Source: CAD feature listing. Evaluate the final solid. Frame: model axes, mm. Face numbers are marked on the shaded views. A direction names the side the tool comes from. Round coordinates to 2 decimals unless told otherwise and drop trailing zeros. Order: outer loops, then holes, each group sorted by start corner. A loop starts at its lowest first (then second) coordinate and runs counter-clockwise, first axis right, second up. Notation, with made-up numbers: (43, 15.25) - (57, 15.25) arc R11 ccw to (57, 23.25) - close; hole circle Ø8 at (3, 75.5). An arc over 180 degrees is marked (long way). Put each result on its own line as item: value. Start each with the question number.
1) Contact query for flat-ended pins moving along their axis: P1, Ø6, axis at x = 68, z = -49.5, coming from the +Y side; P2, Ø4.5, axis at y = -44.5, z = 65, coming from the +X side; P3, Ø5, axis at y = 34, z = 47.5, coming from the -X side; P4, Ø5, axis at x = 10, y = -28, coming from the +Z side. Output: stop coordinate, or through.
2) Line query: probe 1 along Y at (x, z) = (1.5, -30); probe 2 along Y at (x, z) = (90.5, -23.5); probe 3 along Z at (x, y) = (1, -51). Output: solid intervals per line, ascending. Write a range as [from, to].
3) Section A-A on x = -7. Output: boundary loops of the cut face in (y, z).
4) Section B-B on z = 0. Output: boundary loops of the cut face in (x, y).
5) Section D-D on x = 38.5. Output: boundary loops of the cut face in (y, z), then the cut area to 3 significant figures.
6) Access query for the marked faces 4, 5 and 6. Directions: +Z, -Z, +X, -X, +Y, -Y. A direction counts if a zero-diameter tool reaches every point of the face in a straight line with its end or side. Return the directions, or none.
7) Section C-C on z = -21. Output: boundary loops of the cut face in (x, y), then the cut area to 3 significant figures.
8) Mould query, pull axis Z, two halves, no side actions, for the marked faces 1, 2 and 3. Classes: +Z half, -Z half, draft (parallel to the pull), parting line (faces both ways), or undercut.
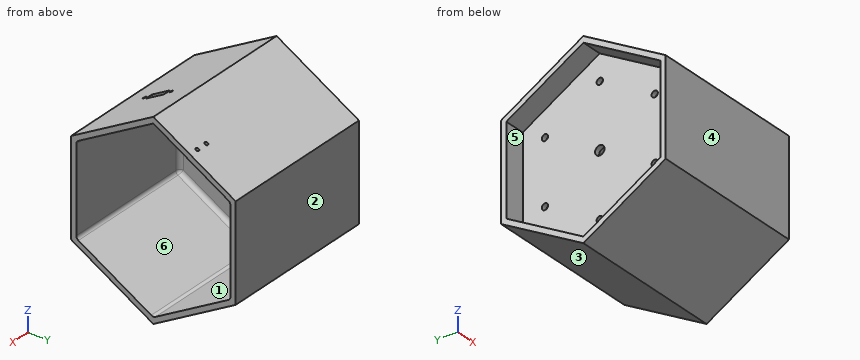
```python
from build123d import *

# Parameters (mm, degrees)
BOSS_EXTRUDE1_DEPTH = 200
CUT_EXTRUDE1_DEPTH  = 195
SKETCH5_R           = 1.65
SKETCH5_W           = 7.65
SKETCH5_H           = 20.2
CUT_EXTRUDE4_DEPTH  = 70
SKETCH7_R           = 4.5
SKETCH7_R_2         = 3
CUT_EXTRUDE6_DEPTH  = 70
FILLET1_R           = 4
CUT_EXTRUDE7_DEPTH  = 70
SKETCH10_R          = 1.6
CUT_EXTRUDE8_DEPTH  = 6
BOSS_EXTRUDE2_DEPTH = 20


with BuildPart() as part:
    # Sketch1 → Boss-Extrude1 (new body)
    with BuildSketch(Plane(origin=(0, 0, 0), x_dir=(0, 0, -1), z_dir=(1, 0, 0))):
        Polygon((90, 0), (45, 77.942286341), (-45, 77.942286341), (-90, 0), (-45, -77.942286341), (45, -77.942286341), align=None)
    extrude(amount=BOSS_EXTRUDE1_DEPTH)

    # Sketch2 → Cut-Extrude1 (cut)
    with BuildSketch(Plane(origin=(200, 0, 0), x_dir=(0, 0, -1), z_dir=(1, 0, 0))):
        Polygon((84.226497308, 0), (42.113248654, 72.942286341), (-42.113248654, 72.942286341), (-84.226497308, 0), (-42.113248654, -72.942286341), (42.113248654, -72.942286341), align=None)
    extrude(amount=-CUT_EXTRUDE1_DEPTH, mode=Mode.SUBTRACT)

    # Sketch5 → Cut-Extrude4 (cut)
    with BuildSketch(Plane(origin=(0, -38.97114317, 67.5), x_dir=(1, 0, 0), z_dir=(0, -0.500000000000007, 0.8660254037844347))):
        with Locations(Location((68.825, 9.75, 0), (0, 0, 270))):
            Circle(SKETCH5_R)
        with Locations(Location((68.825, -19.75, 0), (0, 0, 270))):
            Circle(SKETCH5_R)
        with Locations((68.825, -5)):
            Rectangle(SKETCH5_W, SKETCH5_H)
    extrude(amount=-CUT_EXTRUDE4_DEPTH, mode=Mode.SUBTRACT)

    # Sketch7 → Cut-Extrude6 (cut)
    with BuildSketch(Plane(origin=(5, 0, 0), x_dir=(0, 0, -1), z_dir=(1, 0, 0))):
        Circle(SKETCH7_R)
        with Locations((60, 0)):
            Circle(SKETCH7_R_2)
        with Locations((30, 51.961524227)):
            Circle(SKETCH7_R_2)
        with Locations((-30, 51.961524227)):
            Circle(SKETCH7_R_2)
        with Locations((-60, 0)):
            Circle(SKETCH7_R_2)
        with Locations((-30, -51.961524227)):
            Circle(SKETCH7_R_2)
        with Locations((30, -51.961524227)):
            Circle(SKETCH7_R_2)
    extrude(amount=-CUT_EXTRUDE6_DEPTH, mode=Mode.SUBTRACT)

    # Fillet1
    fillet1_edges = [part.edges().sort_by_distance(p)[0] for p in [
        (5, -36.47114317, -63.169872981),
        (102.5, 0, -84.226497308),
        (5, -72.942286341, 0),
        (102.5, -72.942286341, -42.113248654),
        (5, -36.47114317, 63.169872981),
        (102.5, -72.942286341, 42.113248654),
        (5, 36.47114317, 63.169872981),
        (5, 72.942286341, 0),
        (102.5, 72.942286341, 42.113248654),
        (5, 36.47114317, -63.169872981),
        (102.5, 72.942286341, -42.113248654),
    ]]
    fillet(fillet1_edges, radius=FILLET1_R)

    # Sketch9 → Cut-Extrude7 (cut)
    with BuildSketch(Plane(origin=(200, 0, 0), x_dir=(0, 0, -1), z_dir=(1, 0, 0))):
        Polygon((45, 77.942286341), (90, 0), (45, -77.942286341), (-45, -77.942286341), (-90, 0), (-45, 77.942286341), align=None)
    extrude(amount=-CUT_EXTRUDE7_DEPTH, mode=Mode.SUBTRACT)

    # Sketch10 → Cut-Extrude8 (cut)
    with BuildSketch(Plane(origin=(0, 38.97114317, 67.5), x_dir=(1, 0, 0), z_dir=(0, 0.49999999999999495, 0.8660254037844417))):
        with Locations(Location((110, -5, 0), (0, 0, 270))):
            Circle(SKETCH10_R)
        with Locations(Location((121, -5, 0), (0, 0, 270))):
            Circle(SKETCH10_R)
    extrude(amount=-CUT_EXTRUDE8_DEPTH, mode=Mode.SUBTRACT)

    # Sketch11 → Boss-Extrude2 (add)
    with BuildSketch(Plane.ZY):
        Polygon((90, 0), (45, 77.942286341), (-45, 77.942286341), (-90, 0), (-45, -77.942286341), (45, -77.942286341), align=None)
        Polygon((84.226497308, 0), (42.113248654, 72.942286341), (-42.113248654, 72.942286341), (-84.226497308, 0), (-42.113248654, -72.942286341), (42.113248654, -72.942286341), align=None, mode=Mode.SUBTRACT)
    extrude(amount=BOSS_EXTRUDE2_DEPTH)


solid = part.part
```
Answer sheet:
1. P1: y = 75.34
1. P2: x = 130
1. P3: x = 0
1. P4: z = 75.28
2. probe 1: [-77.94, -54.96], [-48.96, 48.96], [54.96, 77.94]
2. probe 2: [-77.94, -72.94], [72.94, 77.94]
2. probe 3: [-60.56, -32.84], [-27.16, 27.16], [32.84, 60.56]
3. outline: (-77.94, -45) - (0, -90) - (77.94, -45) - (77.94, 45) - (0, 90) - (-77.94, 45) - close; hole (-72.94, -42.11) - (0, -84.23) - (72.94, -42.11) - (72.94, 42.11) - (0, 84.23) - (-72.94, 42.11) - close
4. outline: (-20, -77.94) - (130, -77.94) - (130, -72.94) - (9, -72.94) arc R4 cw to (5, -68.94) - (5, -4.5) - (0, -4.5) - (0, -72.94) - (-20, -72.94) - close; (-20, 72.94) - (0, 72.94) - (0, 4.5) - (5, 4.5) - (5, 68.94) arc R4 cw to (9, 72.94) - (130, 72.94) - (130, 77.94) - (-20, 77.94) - close
5. outline: (-77.94, -45) - (0, -90) - (77.94, -45) - (77.94, 45) - (0, 90) - (-77.94, 45) - close; hole (-72.94, -39.8) arc R4 ccw to (-70.94, -43.27) - (-2, -83.07) arc R4 ccw to (2, -83.07) - (70.94, -43.27) arc R4 ccw to (72.94, -39.8) - (72.94, 39.8) arc R4 ccw to (70.94, 43.27) - (0, 84.23) - (-70.94, 43.27) arc R4 ccw to (-72.94, 39.8) - close
5. area: 2,620 mm^2
6. face 4: +Z, -Z, +X, -X, -Y
6. face 5: -X
6. face 6: +X
7. outline: (-20, -77.94) - (130, -77.94) - (130, -72.94) - (9, -72.94) arc R4 cw to (5, -68.94) - (5, 68.94) arc R4 cw to (9, 72.94) - (130, 72.94) - (130, 77.94) - (-20, 77.94) - (-20, 72.94) - (0, 72.94) - (0, -72.94) - (-20, -72.94) - close
7. area: 2,240 mm^2
8. face 1: undercut
8. face 2: draft
8. face 3: -Z half
